Read the model definition and answer for the solid it produces. Units are mm, in the model's axes. Face numbers are marked on the shaded views. A direction names the side the tool comes from. Coordinates: 2 decimals unless noted, no trailing zeros. Loops run counter-clockwise (first coordinate to the right, second up) from the corner with the lowest first, then second, coordinate; pieces in that order, holes last.
from build123d import *

# Parameters (mm, degrees)
FIVE_MM_ATTACHMENT_FOOT_START                    = -5
SKETCH1_W                                        = 20
SKETCH1_H                                        = 9.5
SKETCH1_R                                        = 1.7
FIVE_MM_ATTACHMENT_FOOT_DEPTH                    = 5
DEEP_ACTUATOR_WEB_START                          = -69
SKETCH2_W                                        = 12
SKETCH2_H                                        = 24
DEEP_ACTUATOR_WEB_DEPTH                          = 67.5
QUARTER20_AXIAL_THREAD_MAJOR_ENVELOPE_DEPTH      = 90.516758208
QUARTER20_AXIAL_THREAD_MAJOR_ENVELOPE_DEPTH_BACK = 90.516758208
SKETCH3_R                                        = 3.175


with BuildPart() as part:
    # Sketch1 → Five_mm_Attachment_Foot (new body)
    with BuildSketch(Plane.XY.offset(FIVE_MM_ATTACHMENT_FOOT_START)):
        with Locations((-20, 29.25)):
            Rectangle(SKETCH1_W, SKETCH1_H)
        with Locations((-27, 28)):
            Circle(SKETCH1_R, mode=Mode.SUBTRACT)
        with Locations((-13, 28)):
            Circle(SKETCH1_R, mode=Mode.SUBTRACT)
    extrude(amount=FIVE_MM_ATTACHMENT_FOOT_DEPTH)

    # Sketch2 → Deep_Actuator_Web (add)
    with BuildSketch(Plane.XY.offset(DEEP_ACTUATOR_WEB_START)):
        with Locations((-20, 36.5)):
            Rectangle(SKETCH2_W, SKETCH2_H)
    extrude(amount=DEEP_ACTUATOR_WEB_DEPTH)

    # Sketch3 → Quarter20_Axial_Thread_Major_Envelope (cut, two sides: drawn at the far end of the back side and taken through both)
    with BuildSketch(Plane(origin=(0, 0, 0), x_dir=(0, 0, -1), z_dir=(1, 0, 0)).offset(-QUARTER20_AXIAL_THREAD_MAJOR_ENVELOPE_DEPTH_BACK)):
        with Locations((69, 36.5)):
            Circle(SKETCH3_R)
    extrude(amount=QUARTER20_AXIAL_THREAD_MAJOR_ENVELOPE_DEPTH + QUARTER20_AXIAL_THREAD_MAJOR_ENVELOPE_DEPTH_BACK, mode=Mode.SUBTRACT)


solid = part.part
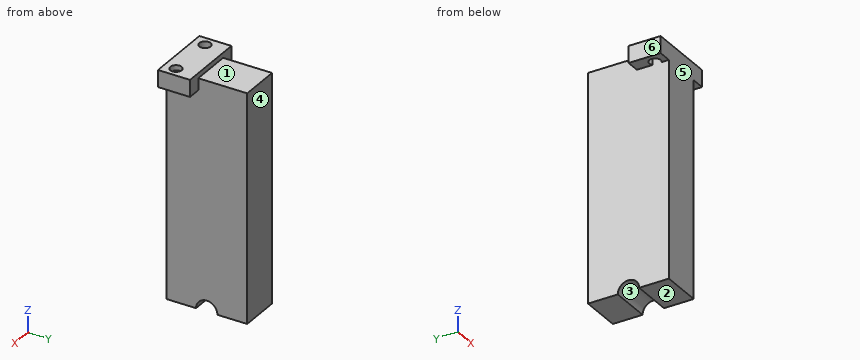
Item 1: A cutting plane is placed at A-A on x = -13. Determine the outline of the cut face in (y, z), then the cut area to 3 significant figures.
Numbers:
outline: (24.5, -5) - (26.3, -5) - (26.3, 0) - (24.5, 0) - close; (29.7, -5) - (34, -5) - (34, 0) - (29.7, 0) - close
area: 30.5 mm2
Item 2: A cutting plane is placed at D-D on z = -53. Determine the outline of the cut face in (x, y), then the cut area to 3 significant figures.
Numbers:
outline: (-26, 24.5) - (-14, 24.5) - (-14, 48.5) - (-26, 48.5) - close
area: 288 mm2
Item 3: A cutting plane is placed at B-B on y = 28. Determine the outline of the cut face in (x, z), then the cut area to 3 significant figures.
Numbers:
outline: (-30, -5) - (-28.7, -5) - (-28.7, 0) - (-30, 0) - close; (-26, -69) - (-14, -69) - (-14, -1.5) - (-14.7, -1.5) - (-14.7, 0) - (-25.3, 0) - (-25.3, -1.5) - (-26, -1.5) - close; (-11.3, -5) - (-10, -5) - (-10, 0) - (-11.3, 0) - close
area: 839 mm2
Item 4: Which of the six approach directions +Z, -Z, +X, -X, +Y, -Y give full straight-line access (tool end or side, diameter ignored) to the marked faces 1 and 2?
Numbers:
face 1: +Z, +X, -X, +Y
face 2: -Z, +X, -X, +Y, -Y
Item 5: A cutting plane is placed at C-C on x = -20. Determine the outline of the cut face in (y, z) (3 decimals).
Numbers:
outline: (24.5, -69) - (33.325, -69) arc R3.175 cw to (39.675, -69) - (48.5, -69) - (48.5, -1.5) - (34, -1.5) - (34, 0) - (24.5, 0) - close
Item 6: Determine the mould class of the marked faces 3, 4, 5 and 6 for opening direction Y: released by +Y, released by -Y, zero draft, split by the parting line, or undercut.
Numbers:
face 3: undercut
face 4: released by +Y
face 5: released by -Y
face 6: zero draft
Item 7: Given pin 1 (6 mm diameter, centred on y = 28, z = -47, fed in from -X); pin 2 (4.5 mm diameter, centred on x = -29, y = 31.5, fed in from -Z); pin 3 (1 mm diameter, centred on x = -27, y = 40, fed in from +Z); pin 4 (9.5 mm diameter, centred on x = -22, y = 42.5, fed in from +Z), each flat-ended and moving along its own axis, determine where each tip first touches the part or whether it passes through.
Numbers:
pin 1: stops at x = -26
pin 2: stops at z = -5
pin 3: passes through
pin 4: stops at z = -1.5
Item 8: Find the intervals of material crossed by line 1 along X through (y, z) = (28, -2.2); line 2 along Y through (x, z) = (-13, -3.3); line 3 along X through (y, z) = (40.25, -47.5), in increasing order.
Numbers:
line 1: x = -30 to -28.7, -26 to -14, -11.3 to -10
line 2: y = 24.5 to 26.3, 29.7 to 34
line 3: x = -26 to -14
